from build123d import *

# Parameters (mm, degrees)
SKETCH1_W           = 53.975
SKETCH1_H           = 69.85
BOSS_EXTRUDE1_DEPTH = 1.5
SKETCH1_4_W         = 56.975
SKETCH1_4_H         = 72.85
SKETCH1_4_W_2       = 53.975
SKETCH1_4_H_2       = 69.85
BOSS_EXTRUDE2_DEPTH = 16.5
CUT_EXTRUDE1_REACH  = 84.822
SKETCH2_W           = 16.55
SKETCH2_H           = 14.5
SKETCH2_W_2         = 15.105
CUT_EXTRUDE2_REACH  = 64.928
SKETCH3_R           = 1.75


with BuildPart() as part:
    # Sketch1 → Boss-Extrude1 (new body)
    with BuildSketch(Plane(origin=(0, 0, 0), x_dir=(1, 0, 0), z_dir=(0, 1, 0))):
        with Locations((7.2918379, -12.641495434)):
            Rectangle(SKETCH1_W, SKETCH1_H)
    extrude(amount=BOSS_EXTRUDE1_DEPTH)

    # Sketch1_4 → Boss-Extrude2 (add)
    with BuildSketch(Plane(origin=(0, 0, 0), x_dir=(1, 0, 0), z_dir=(0, 1, 0))):
        with Locations((7.2918379, -12.641495434)):
            Rectangle(SKETCH1_4_W, SKETCH1_4_H)
        with Locations((7.2918379, -12.641495434)):
            Rectangle(SKETCH1_4_W_2, SKETCH1_4_H_2, mode=Mode.SUBTRACT)
    extrude(amount=BOSS_EXTRUDE2_DEPTH)

    # Sketch2 → Cut-Extrude1 (cut, up to next)
    with BuildSketch(Plane(origin=(0, 0, -23.783504566), x_dir=(-1, 0, 0), z_dir=(0, 0, -1)), mode=Mode.PRIVATE) as cut_extrude1_sk1:
        with Locations((-25.0043379, 9.25)):
            Rectangle(SKETCH2_W, SKETCH2_H)
    cut_extrude1_tool1 = extrude(cut_extrude1_sk1.sketch, amount=-CUT_EXTRUDE1_REACH, mode=Mode.PRIVATE) & part.part
    # Sketch2 → Cut-Extrude1 (cut, up to next)
    with BuildSketch(Plane(origin=(0, 0, -23.783504566), x_dir=(-1, 0, 0), z_dir=(0, 0, -1)), mode=Mode.PRIVATE) as cut_extrude1_sk2:
        with Locations((11.1431621, 9.25)):
            Rectangle(SKETCH2_W_2, SKETCH2_H)
    cut_extrude1_tool2 = extrude(cut_extrude1_sk2.sketch, amount=-CUT_EXTRUDE1_REACH, mode=Mode.PRIVATE) & part.part
    add(cut_extrude1_tool1.solids().sort_by_distance((25.004338, 9.25, -23.783505))[0], mode=Mode.SUBTRACT)
    add(cut_extrude1_tool2.solids().sort_by_distance((-11.143162, 9.25, -23.783505))[0], mode=Mode.SUBTRACT)

    # Sketch3 → Cut-Extrude2 (cut, up to next)
    with BuildSketch(Plane.XZ, mode=Mode.PRIVATE) as cut_extrude2_sk1:
        with Locations(Location((16.8043379, 24.066495434, 0), (0, 0, 270))):
            Circle(SKETCH3_R)
    cut_extrude2_tool1 = extrude(cut_extrude2_sk1.sketch, amount=-CUT_EXTRUDE2_REACH, mode=Mode.PRIVATE) & part.part
    # Sketch3 → Cut-Extrude2 (cut, up to next)
    with BuildSketch(Plane.XZ, mode=Mode.PRIVATE) as cut_extrude2_sk2:
        with Locations(Location((-4.6956621, 24.066495434, 0), (0, 0, 270))):
            Circle(SKETCH3_R)
    cut_extrude2_tool2 = extrude(cut_extrude2_sk2.sketch, amount=-CUT_EXTRUDE2_REACH, mode=Mode.PRIVATE) & part.part
    # Sketch3 → Cut-Extrude2 (cut, up to next)
    with BuildSketch(Plane.XZ, mode=Mode.PRIVATE) as cut_extrude2_sk3:
        with Locations(Location((16.8043379, 6.066495434, 0), (0, 0, 270))):
            Circle(SKETCH3_R)
    cut_extrude2_tool3 = extrude(cut_extrude2_sk3.sketch, amount=-CUT_EXTRUDE2_REACH, mode=Mode.PRIVATE) & part.part
    # Sketch3 → Cut-Extrude2 (cut, up to next)
    with BuildSketch(Plane.XZ, mode=Mode.PRIVATE) as cut_extrude2_sk4:
        with Locations(Location((-4.6956621, 6.066495434, 0), (0, 0, 270))):
            Circle(SKETCH3_R)
    cut_extrude2_tool4 = extrude(cut_extrude2_sk4.sketch, amount=-CUT_EXTRUDE2_REACH, mode=Mode.PRIVATE) & part.part
    add(cut_extrude2_tool1.solids().sort_by_distance((16.804338, 0, 24.066495))[0], mode=Mode.SUBTRACT)
    add(cut_extrude2_tool2.solids().sort_by_distance((-4.695662, 0, 24.066495))[0], mode=Mode.SUBTRACT)
    add(cut_extrude2_tool3.solids().sort_by_distance((16.804338, 0, 6.066495))[0], mode=Mode.SUBTRACT)
    add(cut_extrude2_tool4.solids().sort_by_distance((-4.695662, 0, 6.066495))[0], mode=Mode.SUBTRACT)


solid = part.part
Build history of the part. All positions in model axes, mm. A direction names the side the tool comes from. Give positions to 0.01 mm unless a question says otherwise; leave off trailing zeros. Order: outer loops, then holes, each group sorted by start corner. A loop starts at its lowest first (then second) coordinate and runs counter-clockwise, first axis right, second up. Notation, with made-up numbers: M -32.75,29.25 L -1.75,29.25 A30 ccw -1.75,65.25 Z; hole C 39.5,44 d8. An arc over 180 degrees is marked long. Put each result on its own line as item: value.
Item 1: Drop flat-ended pins along their axis: pin 1 Ø1.2 at (x, z) = (25, -23) entering from +Y; pin 2 Ø1 at (x, z) = (4.5, -4) entering from +Y; pin 3 Ø3 at (x, z) = (25, 13) entering from -Y. Give the stop position or say it passes through.
Results are:
pin 1: y = 2
pin 2: y = 1.5
pin 3: y = 0
Item 2: Cut at A-A on y = 10. Write the cut outline in (x, z).
Results are:
outline: M -21.2,-23.78 L -18.7,-23.78 L -18.7,-22.28 L -19.7,-22.28 L -19.7,47.57 L 34.28,47.57 L 34.28,-22.28 L 33.28,-22.28 L 33.28,-23.78 L 35.78,-23.78 L 35.78,49.07 L -21.2,49.07 Z; M -3.59,-23.78 L 16.73,-23.78 L 16.73,-22.28 L -3.59,-22.28 Z
Item 3: Which spindle directions (+Z, -Z, +X, -X, +Y, -Y) get a long thin tool onto all of the face, cutting with end or side? Do faces 1 (the face through (-11, 2, -23)), 2 (the face through (-19.696, 9, 13)), 3 (the face through (-4.619, 0.74, 7.815)). Say none if no direction does.
Results are:
face 1: -Z, +Y
face 2: +Y
face 3: +Y, -Y
Item 4: Pull direction Z, two halves, no side cores. Call faces 4 (the face through (-3.591, 9, -23)), 5 (the face through (7, 1.5, 12)), 6 (the face through (7, 6, -23.784)), 7 (the face through (3, 8, -22.284)): +Z half, -Z half, draft (parallel to the pull), parting line (faces both ways), or undercut.
Results are:
face 4: draft
face 5: undercut
face 6: -Z half
face 7: undercut
Item 5: Cut at D-D on z = 7. Write the cut outline in (x, y).
Results are:
outline: M -21.2,0 L -6.18,0 L -6.18,1.5 L -19.7,1.5 L -19.7,16.5 L -21.2,16.5 Z; M -3.22,0 L 15.32,0 L 15.32,1.5 L -3.22,1.5 Z; M 18.28,0 L 35.78,0 L 35.78,16.5 L 34.28,16.5 L 34.28,1.5 L 18.28,1.5 Z
Item 6: Cut at C-C on x = -12.5. Write the cut outline in (y, z), then the cut area to 3 significant figures.
Results are:
outline: M 0,-23.78 L 2,-23.78 L 2,-22.28 L 1.5,-22.28 L 1.5,47.57 L 16.5,47.57 L 16.5,49.07 L 0,49.07 Z
area: 133 mm2
Item 7: Cut at B-B on z = 42.5. Write the cut outline in (x, y), then the cut area to 3 significant figures.
Results are:
outline: M -21.2,0 L 35.78,0 L 35.78,16.5 L 34.28,16.5 L 34.28,1.5 L -19.7,1.5 L -19.7,16.5 L -21.2,16.5 Z
area: 130 mm2
Item 8: Wall check: probe 1 along X at (y, z) = (11.75, 41); probe 2 along Z at (x, y) = (11, 11.5); probe 3 along Y at (x, z) = (3, 25). Give the ranges that are in metal, low to high.
Results are:
probe 1: -21.2 to -19.7, 34.28 to 35.78
probe 2: -23.78 to -22.28, 47.57 to 49.07
probe 3: 0 to 1.5
